```python
from build123d import *

# Parameters (mm, degrees)
SKETCH_2_R                   = 4
SKETCH_2_R_2                 = 1.7
EXTRUDE_1_DEPTH              = 6
PATTERN_LINEAR_1_COUNT       = 4
PATTERN_LINEAR_1_PITCH       = 12.5
EXTRUDE_START                = -43.5
SKETCH_3_W                   = 25
SKETCH_3_H                   = 2.5
EXTRUDE_2_DEPTH              = 43.5
SKETCH_4_R                   = 5.5
CUT_EXTRUDE_1_DEPTH          = 6.5
PATTERN_LINEAR_2_COUNT       = 4
PATTERN_LINEAR_2_PITCH       = 12.5
PATTERN_START                = 12.5
PATTERN_LINEAR_3_OUTLINE_R   = 1.7
PATTERN_LINEAR_3_DEPTH       = 6
PATTERN_START_2              = 25
PATTERN_LINEAR_3_2_OUTLINE_R = 1.7
PATTERN_LINEAR_3_2_DEPTH     = 6
PATTERN_START_3              = 37.5
PATTERN_LINEAR_3_3_OUTLINE_R = 1.7
PATTERN_LINEAR_3_3_DEPTH     = 6
MIRROR_3_COPY_1_SKETCH_R     = 5.5
MIRROR_3_COPY_1_DEPTH        = 6.5
MIRROR_3_COPY_2_SKETCH_R     = 5.5
MIRROR_3_COPY_2_DEPTH        = 6.5
MIRROR_3_COPY_3_SKETCH_R     = 5.5
MIRROR_3_COPY_3_DEPTH        = 6.5
SKETCH_5_W                   = 3
SKETCH_5_H                   = 14
SKETCH_5_H_2                 = 19
EXTRUDE_3_DEPTH              = 6
SKETCH_6_R                   = 4
EXTRUDE_4_DEPTH              = 6
CUT_EXTRUDE_2_DEPTH          = 20
CUT_EXTRUDE_2_DEPTH_BACK     = 10
SKETCH_7_R                   = 1.6
CHAMFER_1_SIZE               = 2
CHAMFER_2_SIZE               = 1.81151278


with BuildPart() as part:
    # Sketch 2 → Extrude 1 (new body)
    with BuildSketch(Plane.XY):
        Circle(SKETCH_2_R)
        Circle(SKETCH_2_R_2, mode=Mode.SUBTRACT)
    extrude_1 = extrude(amount=EXTRUDE_1_DEPTH)


with BuildPart() as pattern_linear_1_1:
    # Pattern Linear 1: pattern copy
    add(part.part.moved(Location(Vector(0, 0, 1) * (1 * PATTERN_LINEAR_1_PITCH))))


with BuildPart() as pattern_linear_1_2:
    # Pattern Linear 1: pattern copy
    add(part.part.moved(Location(Vector(0, 0, 1) * (2 * PATTERN_LINEAR_1_PITCH))))


with BuildPart() as pattern_linear_1_3:
    # Pattern Linear 1: pattern copy
    add(part.part.moved(Location(Vector(0, 0, 1) * (3 * PATTERN_LINEAR_1_PITCH))))


with BuildPart() as part_1:
    add(part.part)

    add(pattern_linear_1_1.part)  # Extrude 2 merges Pattern Linear 1_1

    add(pattern_linear_1_2.part)  # Extrude 2 merges Pattern Linear 1_2

    add(pattern_linear_1_3.part)  # Extrude 2 merges Pattern Linear 1_3
    # Sketch 3 → Extrude 2 (add)
    with BuildSketch(Plane(origin=(0, 0, 0), x_dir=(-1, 0, 0), z_dir=(0, 0, -1)).offset(EXTRUDE_START)):
        with Locations((16.299671038, 0)):
            Rectangle(SKETCH_3_W, SKETCH_3_H)
    extrude(amount=EXTRUDE_2_DEPTH)

    # Sketch 4 → Cut-Extrude 1 (cut)
    with BuildSketch(Plane.XY.offset(6)):
        Circle(SKETCH_4_R)
    cut_extrude_1 = extrude(amount=CUT_EXTRUDE_1_DEPTH, mode=Mode.SUBTRACT)

    # Pattern Linear 2: Cut-Extrude 1 ×4
    with Locations(*[(0, 0, i * PATTERN_LINEAR_2_PITCH) for i in range(1, PATTERN_LINEAR_2_COUNT)]):
        add(cut_extrude_1, mode=Mode.SUBTRACT)

    # Mirror 1: Extrude 1 across plane
    add(extrude_1.mirror(Plane.ZY.offset(16.299671038)))

    # Pattern Linear 3: read off the stored shape, not the designer's step
    # Pattern Linear 3 outline → Pattern Linear 3 (add)
    with BuildSketch(Plane.XY.offset(PATTERN_START)):
        with BuildLine():
            ThreePointArc((-28.799671038, 1.25), (-36.599342077, 0), (-28.799671038, -1.25))
            Line((-28.799671038, -1.25), (-28.799671038, 1.25))
        make_face()
        with Locations((-32.599342077, 0)):
            Circle(PATTERN_LINEAR_3_OUTLINE_R, mode=Mode.SUBTRACT)
    extrude(amount=PATTERN_LINEAR_3_DEPTH)

    # Pattern Linear 3 2 outline → Pattern Linear 3 2 (add)
    with BuildSketch(Plane.XY.offset(PATTERN_START_2)):
        with BuildLine():
            ThreePointArc((-28.799671038, 1.25), (-36.599342077, 0), (-28.799671038, -1.25))
            Line((-28.799671038, -1.25), (-28.799671038, 1.25))
        make_face()
        with Locations((-32.599342077, 0)):
            Circle(PATTERN_LINEAR_3_2_OUTLINE_R, mode=Mode.SUBTRACT)
    extrude(amount=PATTERN_LINEAR_3_2_DEPTH)

    # Pattern Linear 3 3 outline → Pattern Linear 3 3 (add)
    with BuildSketch(Plane.XY.offset(PATTERN_START_3)):
        with BuildLine():
            ThreePointArc((-28.799671038, 1.25), (-36.599342077, 0), (-28.799671038, -1.25))
            Line((-28.799671038, -1.25), (-28.799671038, 1.25))
        make_face()
        with Locations((-32.599342077, 0)):
            Circle(PATTERN_LINEAR_3_3_OUTLINE_R, mode=Mode.SUBTRACT)
    extrude(amount=PATTERN_LINEAR_3_3_DEPTH)

    # Mirror 3: Cut-Extrude 1 across plane
    add(cut_extrude_1.mirror(Plane.ZY.offset(16.299671038)), mode=Mode.SUBTRACT)

    # Mirror 3 copy 1 sketch → Mirror 3 copy 1 (cut)
    with BuildSketch(Plane(origin=(-32.599342077, 0, 18.5), x_dir=(-1, 0, 0), z_dir=(0, 0, 1))):
        Circle(MIRROR_3_COPY_1_SKETCH_R)
    extrude(amount=MIRROR_3_COPY_1_DEPTH, mode=Mode.SUBTRACT)

    # Mirror 3 copy 2 sketch → Mirror 3 copy 2 (cut)
    with BuildSketch(Plane(origin=(-32.599342077, 0, 31), x_dir=(-1, 0, 0), z_dir=(0, 0, 1))):
        Circle(MIRROR_3_COPY_2_SKETCH_R)
    extrude(amount=MIRROR_3_COPY_2_DEPTH, mode=Mode.SUBTRACT)

    # Mirror 3 copy 3 sketch → Mirror 3 copy 3 (cut)
    with BuildSketch(Plane(origin=(-32.599342077, 0, 43.5), x_dir=(-1, 0, 0), z_dir=(0, 0, 1))):
        Circle(MIRROR_3_COPY_3_SKETCH_R)
    extrude(amount=MIRROR_3_COPY_3_DEPTH, mode=Mode.SUBTRACT)

    # Sketch 5 → Extrude 3 (add)
    with BuildSketch(Plane(origin=(0, 0, 12.5), x_dir=(-1, 0, 0), z_dir=(0, 0, -1))):
        with Locations((32.599342077, 10.708099244)):
            Rectangle(SKETCH_5_W, SKETCH_5_H)
        with Locations((15.599342077, 10.75)):
            Rectangle(SKETCH_5_W, SKETCH_5_H_2)
    extrude_3 = extrude(amount=-EXTRUDE_3_DEPTH)

    # Mirror 4: Extrude 3 across plane
    add(extrude_3.mirror(Plane.XY.offset(21.75)))

    # Sketch 6 → Extrude 4 (add)
    with BuildSketch(Plane(origin=(0, 0, 25), x_dir=(-1, 0, 0), z_dir=(0, 0, -1))):
        with Locations((32.599342077, 17.708099244)):
            Circle(SKETCH_6_R)
        with Locations((15.599342077, 20.25)):
            Circle(SKETCH_6_R)
    extrude_4 = extrude(amount=-EXTRUDE_4_DEPTH)

    # Mirror 5: Extrude 4 across plane
    add(extrude_4.mirror(Plane.XY.offset(21.75)))

    # Sketch 7 → Cut-Extrude 2 (cut, two sides: drawn at the far end of the back side and taken through both)
    with BuildSketch(Plane(origin=(0, 0, 25), x_dir=(-1, 0, 0), z_dir=(0, 0, -1)).offset(-CUT_EXTRUDE_2_DEPTH_BACK)):
        with Locations(Location((32.599342077, 17.708099244, 0), (0, 0, 180))):
            Circle(SKETCH_7_R)
        with Locations(Location((15.599342077, 20.25, 0), (0, 0, 180))):
            Circle(SKETCH_7_R)
    extrude(amount=CUT_EXTRUDE_2_DEPTH + CUT_EXTRUDE_2_DEPTH_BACK, mode=Mode.SUBTRACT)

    # Chamfer 1
    chamfer_1_edges = [part_1.edges().sort_by_distance(p)[0] for p in [
        (-14.099342077, 1.25, 15.5),
        (-17.099342077, 1.25, 15.5),
        (-14.099342077, 1.25, 28),
        (-17.099342077, 1.25, 28),
    ]]
    chamfer(chamfer_1_edges, length=CHAMFER_1_SIZE)

    # Chamfer 2
    # the kernel refuses this chamfer: 1.81151278, 1 mm, written as the material it adds along each edge
    with BuildSketch(Plane(origin=(-31.099342077, 3.708099244, 12.5), x_dir=(0, 1, 0), z_dir=(0, 0, 1))) as chamfer_2_piece_1:
        with BuildLine():
            Line((CHAMFER_2_SIZE, 0), (-0.60562029, -1.024801843))
            ThreePointArc((-0.60562029, -1.024801843), (-0.279646114, -0.560511864), (0, 0))
            Line((0, 0), (CHAMFER_2_SIZE, 0))
        make_face()
    extrude(amount=6)
    with BuildSketch(Plane(origin=(-34.099342077, 3.708099244, 12.5), x_dir=(-0.8609060833404796, -0.5087639095566383, 0), z_dir=(0, 0, 1))) as chamfer_2_piece_2:
        with BuildLine():
            Line((1.190375888, 0), (-CHAMFER_2_SIZE * 0.508763909682, -CHAMFER_2_SIZE * 0.860906083552))
            Line((-CHAMFER_2_SIZE * 0.508763909682, -CHAMFER_2_SIZE * 0.860906083552), (0, 0))
            ThreePointArc((0, 0), (0.624821924, -0.044419166), (1.190375888, 0))
        make_face()
    extrude(amount=6)
    with BuildSketch(Plane(origin=(-31.099342077, 3.708099244, 31), x_dir=(0, 1, 0), z_dir=(0, 0, -1))) as chamfer_2_piece_3:
        with BuildLine():
            Line((CHAMFER_2_SIZE, 0), (-0.60562029, 1.024801843))
            ThreePointArc((-0.60562029, 1.024801843), (-0.279646114, 0.560511864), (0, 0))
            Line((0, 0), (CHAMFER_2_SIZE, 0))
        make_face()
    extrude(amount=6)
    with BuildSketch(Plane(origin=(-34.099342077, 3.708099244, 31), x_dir=(-0.8609060833404796, -0.5087639095566383, 0), z_dir=(0, 0, -1))) as chamfer_2_piece_4:
        with BuildLine():
            Line((1.190375888, 0), (-CHAMFER_2_SIZE * 0.508763909682, CHAMFER_2_SIZE * 0.860906083552))
            Line((-CHAMFER_2_SIZE * 0.508763909682, CHAMFER_2_SIZE * 0.860906083552), (0, 0))
            ThreePointArc((0, 0), (0.624821924, 0.044419166), (1.190375888, 0))
        make_face()
    extrude(amount=6)


solid = part_1.part
```
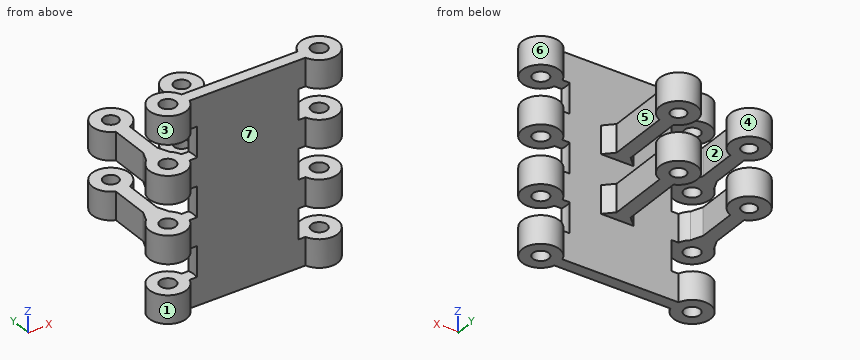
Source: CAD feature listing. Evaluate the final solid. Frame: model axes, mm. Face numbers are marked on the shaded views. A direction names the side the tool comes from. Coordinates: 2 decimals unless noted, no trailing zeros. Loops run counter-clockwise (first coordinate to the right, second up) from the corner with the lowest first, then second, coordinate; pieces in that order, holes last. Notation, with made-up numbers: M 37,-24 L 47,-24 A9 cw 47,-20 Z; hole C 39.25,-21.75 d1. An arc over 180 degrees is marked long. Use CSV: the item, a comma, the result in double quotes.
(1) Cut plane B-B on y = 20.25. Return loops of the section in (x, z), and give its area (3 significant figures).
Answers follow:
outline,"M -35.69,12.5 L -29.51,12.5 L -29.51,18.5 L -35.69,18.5 Z; M -35.69,25 L -29.51,25 L -29.51,31 L -35.69,31 Z; M -19.6,12.5 L -17.2,12.5 L -17.2,18.5 L -19.6,18.5 Z; M -19.6,25 L -17.2,25 L -17.2,31 L -19.6,31 Z; M -14,12.5 L -11.6,12.5 L -11.6,18.5 L -14,18.5 Z; M -14,25 L -11.6,25 L -11.6,31 L -14,31 Z"
area,"132 mm²"
(2) Contact query for flat-ended pins moving along their axis: pin 1 (3 mm diameter, centred on y = 9, z = 28, fed in from -X); pin 2 (20 mm diameter, centred on x = -18, z = 27, fed in from -Y); pin 3 (3 mm diameter, centred on x = -31.5, y = 14, fed in from +Z). Output: stop coordinate, or through.
Answers follow:
pin 1,"x = -34.1"
pin 2,"y = -1.25"
pin 3,"z = 31"
(3) Draft query along Y for the marked faces 4, 5, 6 and 7. Return one class per face: pulls with the +Y half, pulls with the -Y half, needs draft (parallel to the pull), parting line crosses it, or undercut.
Answers follow:
face 4,"undercut"
face 5,"undercut"
face 6,"parting line crosses it"
face 7,"pulls with the -Y half"
(4) Cut plane C-C on z = 5. Return loops of the section in (x, y), and give its area (3 significant figures).
Answers follow:
outline,"M -28.8,-1.25 L -3.8,-1.25 A4 ccw long -3.8,1.25 L -28.8,1.25 A4 ccw long Z; hole C -32.6,0 d3.4; hole C 0,0 d3.4"
area,"144 mm²"
(5) Reachability of the marked faces 1, 2 and 3 from +Z, -Z, +X, -X, +Y, -Y: full face, straight path, thin tool, end or side. Return the list, or none.
Answers follow:
face 1,"-Z"
face 2,"+Z, -Z"
face 3,"+Z"
(6) Cut plane A-A on x = 0. Give the number of separate pieces and of enclosed holes in the cut face, and give its area (3 significant figures).
Answers follow:
separate pieces,"8"
enclosed holes,"0"
area,"110 mm²"
(7) Line query: line 1 (Y direction, x = 0, z = 2.05); line 2 (Z direction, x = -15, y = 22.5); line 3 (Y direction, x = -14.5, z = 41). Output: solid intervals per line, ascending. Write a range as [from, to].
Answers follow:
line 1,"[-4, -1.7], [1.7, 4]"
line 2,"[12.5, 18.5], [25, 31]"
line 3,"[-1.25, 1.25]"
(8) Cut plane D-D on x = -18.5. Return loops of the section in (y, z), and give its area (3 significant figures).
Answers follow:
outline,"M -1.25,0 L 1.25,0 L 1.25,12.5 L 1.85,12.5 L 1.85,18.5 L 1.25,18.5 L 1.25,25 L 1.85,25 L 1.85,31 L 1.25,31 L 1.25,43.5 L -1.25,43.5 Z; M 17.5,12.5 L 23,12.5 L 23,18.5 L 17.5,18.5 Z; M 17.5,25 L 23,25 L 23,31 L 17.5,31 Z"
area,"182 mm²"
